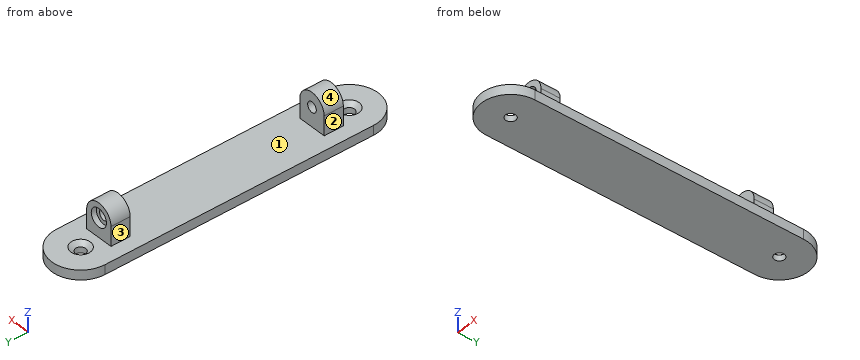
```python
from build123d import *

# Parameters (mm, degrees)
BOSS_EXTRUDE1_DEPTH                                 = 6.35
CSK_FOR_1_4_FLAT_HEAD_MACHINE_SCREW_100_D           = 6.7564
CSK_FOR_1_4_FLAT_HEAD_MACHINE_SCREW_100_CSINK_D     = 12.8778
CSK_FOR_1_4_FLAT_HEAD_MACHINE_SCREW_100_CSINK_ANGLE = 100
SKETCH6_W                                           = 19.05
SKETCH6_H                                           = 12.7
BOSS_EXTRUDE2_DEPTH                                 = 12.7
BOSS_EXTRUDE3_DEPTH                                 = 12.7
CBORE_FOR_1_4_BUTTON_HEAD_CAP_SCREW1_D              = 6.7564
CBORE_FOR_1_4_BUTTON_HEAD_CAP_SCREW1_CBORE_D        = 11.90752
CBORE_FOR_1_4_BUTTON_HEAD_CAP_SCREW1_CBORE_DEPTH    = 3.3528


with BuildPart() as part:
    # Sketch1 → Boss-Extrude1 (new body)
    with BuildSketch(Plane.XY):
        with BuildLine():
            Line((0, 0), (0, 88.9))
            ThreePointArc((0, 88.9), (19.05, 107.95), (38.1, 88.9))
            Line((38.1, 88.9), (38.1, 0))
            Line((38.1, 0), (0, 0))
        make_face()
    extrude(amount=BOSS_EXTRUDE1_DEPTH)

    # CSK for 1/4 Flat Head Machine Screw (100)1 (through all)
    with Locations(Plane.XY.offset(6.35)):
        with Locations((19.05, 88.9)):
            CounterSinkHole(CSK_FOR_1_4_FLAT_HEAD_MACHINE_SCREW_100_D / 2, CSK_FOR_1_4_FLAT_HEAD_MACHINE_SCREW_100_CSINK_D / 2, counter_sink_angle=CSK_FOR_1_4_FLAT_HEAD_MACHINE_SCREW_100_CSINK_ANGLE)

    # Sketch6 → Boss-Extrude2 (add)
    with BuildSketch(Plane.XY.offset(6.35)):
        with Locations((19.05, 70.519259932)):
            Rectangle(SKETCH6_W, SKETCH6_H)
    extrude(amount=BOSS_EXTRUDE2_DEPTH)

    # Sketch10 → Boss-Extrude3 (add)
    with BuildSketch(Plane(origin=(0, 76.869259932, 0), x_dir=(1, 0, 0), z_dir=(0, 1, 0))):
        with BuildLine():
            Line((9.525, -19.05), (28.575, -19.05))
            ThreePointArc((28.575, -19.05), (19.05, -28.575), (9.525, -19.05))
        make_face()
    extrude(amount=-BOSS_EXTRUDE3_DEPTH)

    # CBORE for 1/4 Button Head Cap Screw1 (through all)
    with Locations(Plane(origin=(0, 76.869259932, 0), x_dir=(1, 0, 0), z_dir=(0, 1, 0))):
        with Locations((19.05, -19.05)):
            CounterBoreHole(CBORE_FOR_1_4_BUTTON_HEAD_CAP_SCREW1_D / 2, CBORE_FOR_1_4_BUTTON_HEAD_CAP_SCREW1_CBORE_D / 2, CBORE_FOR_1_4_BUTTON_HEAD_CAP_SCREW1_CBORE_DEPTH)

    # Mirror1: part across plane


with BuildPart() as part_1:
    add(part.part)
    add(part.part.mirror(Plane(origin=(0, 0, 6.35), x_dir=(0, 0, 1), z_dir=(0, 1, 0))))


solid = part_1.part
```
Geometry check sheet. Reference: the model listing, model coordinates, mm. Face numbers are marked on the shaded views. A direction names the side the tool comes from. Coordinates: 2 decimals unless noted, no trailing zeros. Loops run counter-clockwise (first coordinate to the right, second up) from the corner with the lowest first, then second, coordinate; pieces in that order, holes last.
Item 1: Access from +Z, -Z, +X, -X, +Y, -Y to the whole of each face (thin tool, end or side, straight path). Record for the marked faces 3 and 4.
Item 2: Sectioned sample at B-B, the plane x = 19.05. Count the separate pieces of the cut face and the enclosed holes in it, then the cut area to 3 significant figures.
Item 3: Sectioned sample at D-D, the plane x = 35.5. Record the boundary of the cut face in (y, z), then the cut area to 3 significant figures.
Item 4: Release check for a two-part mould opening along Y. For the marked faces 1 and 2 record: released by +Y, released by -Y, zero draft, split by the parting line, or undercut.
Item 5: Sectioned sample at A-A, the plane z = 9. Record the boundary of the cut face in (x, y) (3 decimals), then the cut area to 3 significant figures.
Item 6: Thickness scan on line 1 (Y direction, x = 19.05, z = 2.4); line 2 (Y direction, x = 24, z = 20); line 3 (Z direction, x = 19.05, y = -74.85) (3 decimals). Record the ranges inside material, lowest first.
Item 7: Go/stop test with flat-tipped pins: pin 1 Ø8 at (x, y) = (19.05, -88.9) entering from +Z; pin 2 Ø15.5 at (x, z) = (19.05, 19.05) entering from -Y; pin 3 Ø3 at (x, z) = (19, 11.5) entering from +Y. Record where each tip stops, or that it passes through.
Item 8: Sectioned sample at C-C, the plane y = -10.5. Record the boundary of the cut face in (x, z), then the cut area to 3 significant figures.
Check result:
1. face 3: +Z, -X, +Y, -Y
1. face 4: +Z, +Y, -Y
2. separate pieces: 5
2. enclosed holes: 0
2. area: 1,630 mm2
3. outline: (-98.51, 0) - (98.51, 0) - (98.51, 6.35) - (-98.51, 6.35) - close
3. area: 1,250 mm2
4. face 1: undercut
4. face 2: zero draft
5. outline: (9.525, -76.869) - (28.575, -76.869) - (28.575, -64.169) - (9.525, -64.169) - close; (9.525, 64.169) - (28.575, 64.169) - (28.575, 76.869) - (9.525, 76.869) - close
5. area: 484 mm2
6. line 1: y = -107.95 to -92.28, -85.52 to 85.52, 92.28 to 107.95
6. line 2: y = -73.52 to -64.17, 64.17 to 73.52
6. line 3: z = 0 to 13.096, 25.004 to 28.575
7. pin 1: stops at z = 4.3
7. pin 2: stops at y = -76.87
7. pin 3: stops at y = 76.87
8. outline: (0, 0) - (38.1, 0) - (38.1, 6.35) - (0, 6.35) - close
8. area: 242 mm2
